Autodesk Inventor part; units mm, degrees
ref_plane "YZ Plane" through (0, 0, 0) normal (1, 0, 0) x (0, 1, 0)
ref_plane "XZ Plane" through (0, 0, 0) normal (0, 1, 0) x (-1, 0, 0)
ref_plane "XY Plane" through (0, 0, 0) normal (0, 0, 1) x (1, 0, 0)
sketch "Sketch1" plane through (0, 0, 0) normal (0, 0, 1) x (1, 0, 0)
  line L0 (0, 0) -> (103.9622, 0)
  line L1 (103.9622, 0) -> (103.9622, 50.8)
  line L2 (103.9622, 50.8) -> (0, 50.8)
  line L3 (0, 50.8) -> (0, 0)
  line L4 (0, 50.8) -> (103.9622, 50.8)
  line L5 (103.9622, 50.8) -> (103.9622, 42.9936)
  line L6 (0, 42.9936) -> (0, 50.8)
  dimension "d4" = 103.9622
  dimension "d5" = 50.8
extrude "Extrusion1" add sketch "Sketch1" along normal blind 2.54
sketch "Sketch6" plane through (0, 0, 2.54) normal (0, 0, 1) x (1, 0, 0)
  line L0 (103.9622, 0) -> (103.9622, 50.8)
  line L1 (103.9622, 50.8) -> (0, 50.8)
  line L2 (0, 50.8) -> (0, 0)
  line L3 (0, 0) -> (103.9622, 0)
  line L4 (0, 0) -> (2.54, 0)
  line L5 (2.54, 0) -> (2.54, 50.8)
  line L6 (2.54, 50.8) -> (0, 50.8)
  line L7 (0, 50.8) -> (0, 0)
  dimension "d23" = 2.54
  dimension "d24" = 50.8
extrude "Extrusion5" add sketch "Sketch6" along normal blind 103.9622 contours L3 L2 L1 L5
sketch "Sketch7" plane through (2.54, 0, 2.54) normal (1, 0, 0) x (0, 0, -1)
  line L0 (0, 50.8) -> (0, 0)
  line L1 (0, 50.8) -> (-103.9622, 50.8)
  line L2 (-103.9622, 0) -> (-103.9622, 50.8)
  line L3 (0, 0) -> (-103.9622, 0)
  line L4 (2.54, 0) -> (2.54, 50.8)
  line L5 (2.54, 50.8) -> (0, 50.8)
  line L6 (0, 0) -> (0, 50.8)
  line L7 (2.54, 0) -> (0, 0)
  line L8 (0, 50.8) -> (0, 0)
  line L9 (0, 50.8) -> (-103.9622, 50.8)
  line L10 (-103.9622, 0) -> (-103.9622, 50.8)
  line L11 (0, 0) -> (-103.9622, 0)
  circle A0 centre (-10.2616, 39.1541) radius 1.905
  circle A1 centre (-10.2616, 11.6459) radius 1.905
  circle A2 centre (-54.7116, 39.1541) radius 1.905
  circle A3 centre (-54.7116, 11.6459) radius 1.905
  dimension "d27" = 3.81
  dimension "d28" = 11.6459
  dimension "d29" = 10.2616
  dimension "d30" = 3.81
  dimension "d31" = 11.6459
  dimension "d32" = 3.81
  dimension "d33" = 3.81
  dimension "d34" = 44.45
  dimension "d35" = 44.45
  dimension "d36" = 11.6459
  dimension "d37" = 10.2616
  dimension "d38" = 11.6459
extrude "Extrusion6" cut sketch "Sketch7" against normal through all contours A0 | A1 | A2 | A3
sketch "Sketch8" plane through (0, 0, 2.54) normal (0, 0, 1) x (1, 0, 0)
  circle A0 centre (12.8016, 39.1541) radius 1.905
  circle A1 centre (12.8016, 11.6459) radius 1.905
  circle A2 centre (57.2516, 39.1541) radius 1.905
  circle A3 centre (57.2516, 11.6459) radius 1.905
  line L0 (103.9622, 50.8) -> (2.54, 50.8)
  line L1 (2.54, 0) -> (103.9622, 0)
  line L2 (2.54, 0) -> (2.54, 50.8)
  line L3 (103.9622, 50.8) -> (26.416, 50.8)
  line L4 (26.416, 50.8) -> (26.416, 48.26)
  line L5 (26.416, 48.26) -> (103.9622, 48.26)
  line L6 (103.9622, 48.26) -> (103.9622, 50.8)
  line L7 (2.54, 13.5509) -> (2.54, 9.7409)
  line L8 (2.54, 41.0591) -> (2.54, 37.2491)
  line L9 (2.54, 13.5509) -> (2.54, 9.7409)
  line L10 (2.54, 41.0591) -> (2.54, 37.2491)
  line L11 (2.54, 50.8) -> (2.54, 0)
  line L12 (2.54, 0) -> (2.54, 50.8)
  line L13 (2.54, 13.5509) -> (2.54, 9.7409)
  line L14 (2.54, 41.0591) -> (2.54, 37.2491)
  line L15 (2.54, 13.5509) -> (2.54, 9.7409)
  line L16 (2.54, 41.0591) -> (2.54, 37.2491)
  line L17 (2.54, 50.8) -> (2.54, 0)
  line L18 (2.54, 0) -> (2.54, 50.8)
  point P0 (0, 0)
  dimension "d41" = 3.81
  dimension "d42" = 3.81
  dimension "d43" = 3.81
  dimension "d44" = 3.81
  dimension "d45" = 11.6459
  dimension "d46" = 11.6459
  dimension "d47" = 11.6459
  dimension "d48" = 11.6459
  dimension "d49" = 10.2616
  dimension "d50" = 10.2616
  dimension "d51" = 44.45
  dimension "d52" = 44.45
  dimension "d55" = 77.5462
  dimension "d56" = 2.54
extrude "Extrusion7" cut sketch "Sketch8" against normal through all contours A0 | A1 | A2 | A3
sketch "Sketch9" plane through (2.54, 0, 2.54) normal (1, 0, 0) x (0, 0, -1)
  circle A0 centre (-54.7116, 11.6459) radius 1.905
  circle A1 centre (-54.7116, 39.1541) radius 1.905
  circle A2 centre (-10.2616, 11.6459) radius 1.905
  circle A3 centre (-10.2616, 39.1541) radius 1.905
  line L0 (0, 50.8) -> (0, 0)
  line L1 (0, 50.8) -> (-103.9622, 50.8)
  line L2 (-103.9622, 0) -> (-103.9622, 50.8)
  line L3 (0, 0) -> (-103.9622, 0)
  line L4 (-103.9622, 50.8) -> (-26.416, 50.8)
  line L5 (-26.416, 50.8) -> (-26.416, 48.26)
  line L6 (-26.416, 48.26) -> (-103.9622, 48.26)
  line L7 (-103.9622, 48.26) -> (-103.9622, 50.8)
  point P0 (2.54, 0)
  point P1 (-26.416, 50.8)
  dimension "d57" = 77.5462
  dimension "d58" = 2.54
extrude "Extrusion8" add sketch "Sketch9" along normal blind 16.129 contours L5 L6 L2 L1
sketch "Sketch10" plane through (0, 0, 2.54) normal (0, 0, 1) x (1, 0, 0)
  circle A0 centre (12.8016, 11.6459) radius 1.905
  circle A1 centre (57.2516, 39.1541) radius 1.905
  circle A2 centre (57.2516, 11.6459) radius 1.905
  circle A3 centre (12.8016, 39.1541) radius 1.905
  line L0 (2.54, 50.8) -> (2.54, 0)
  line L1 (2.54, 0) -> (103.9622, 0)
  line L2 (103.9622, 0) -> (103.9622, 50.8)
  line L3 (103.9622, 50.8) -> (2.54, 50.8)
  line L4 (103.9622, 50.8) -> (26.416, 50.8)
  line L5 (26.416, 50.8) -> (26.416, 48.26)
  line L6 (26.416, 48.26) -> (103.9622, 48.26)
  line L7 (103.9622, 48.26) -> (103.9622, 50.8)
  point P0 (0, 0)
  dimension "d61" = 77.5462
  dimension "d62" = 2.54
extrude "Extrusion9" add sketch "Sketch10" along normal blind 16.129 contours L3 L2 L6 L5
sketch "Sketch11" plane through (0, 50.8, 0) normal (0, 1, 0) x (1, 0, 0)
  line L0 (103.9622, 0) -> (0, 0)
  line L1 (0, 0) -> (0, -106.5022)
  line L2 (0, -106.5022) -> (18.669, -106.5022)
  line L3 (18.669, -28.956) -> (18.669, -106.5022)
  line L4 (2.54, -28.956) -> (18.669, -28.956)
  line L5 (2.54, -2.54) -> (2.54, -28.956)
  line L6 (26.416, -2.54) -> (2.54, -2.54)
  line L7 (26.416, -2.54) -> (26.416, -18.669)
  line L8 (103.9622, -18.669) -> (26.416, -18.669)
  line L9 (103.9622, 0) -> (103.9622, -18.669)
  line L10 (15.0876, -28.956) -> (15.0876, -106.5022)
  circle A0 centre (15.0876, -93.8022) radius 2.5019
  circle A1 centre (15.0876, -81.1022) radius 2.5019
  circle A2 centre (15.0876, -68.4022) radius 2.5019
  circle A3 centre (15.0876, -55.7022) radius 2.5019
  circle A4 centre (15.0876, -43.0022) radius 2.5019
  line L11 (26.416, -15.0876) -> (103.9622, -15.0876)
  circle A5 centre (91.2622, -15.0876) radius 2.5019
  circle A6 centre (78.5622, -15.0876) radius 2.5019
  circle A7 centre (65.8622, -15.0876) radius 2.5019
  circle A8 centre (53.1622, -15.0876) radius 2.5019
  circle A9 centre (40.4622, -15.0876) radius 2.5019
  point P0 (0, 0)
  dimension "d65" = 3.5814
  dimension "d66" = 5.0038
  dimension "d67" = 12.7
  dimension "d70" = 12.7
  dimension "d75" = 3.5814
  dimension "d76" = 5.0038
  dimension "d77" = 12.7
  dimension "d80" = 12.7
extrude "Extrusion10" cut sketch "Sketch11" against normal blind 16.129 contours A5 L11 | L11 A5 | A0 L10 | L10 A0 | A6 L11 | L11 A6 | A9 L11 | L11 A9 | A1 L10 | L10 A1 | A7 L11 | L11 A7 | A4 L10 | L10 A4 | A8 L11 | L11 A8 | A2 L10 | L10 A2 | A3 L10 | L10 A3
properties part number "BDVBS_002_Brachet 2" material "Aluminum 6061"
Model file for the job. Use its own axes, mm. A direction names the side the tool comes from. Give positions to 0.01 mm unless a question says otherwise; leave off trailing zeros. Loops run counter-clockwise (first coordinate to the right, second up) from the corner with the lowest first, then second, coordinate; pieces in that order, holes last. Notation, with made-up numbers: (-20.5, -18.5) -> (8.5, -18.5) arc R23 ccw to (8.5, 15.5) -> close; hole circle Ø2 at (-2, 51). An arc over 180 degrees is marked (long way). Write each question's results on one line, items separated by ' | '.
(1) Probe line 1 along X through (y, z) = (27.5, 33); line 2 along Y through (x, z) = (13, 35). List the from-to ranges inside material, lowest first.
Geometry results:
line 1: x = 0 to 2.54 | line 2: y = 48.26 to 50.8
(2) Cut at C-C on x = 23.5. List the corners of the cut face in (y, z).
Geometry results:
outline: (0, 0) -> (50.8, 0) -> (50.8, 2.54) -> (0, 2.54) -> close
(3) Cut at B-B on z = 34. List the corners of the cut face in (x, y), and give its area (3 significant figures).
Geometry results:
outline: (0, 0) -> (2.54, 0) -> (2.54, 48.26) -> (18.67, 48.26) -> (18.67, 50.8) -> (0, 50.8) -> close | area: 170 mm²
(4) Tool access for faces 1 (the cylindrical face through (1.288, 13.535, 13.05)), 2 (the flat face through (18.669, 50, 68)), 3 (the flat face through (65, 48.26, 10)): list every direction of +Z, -Z, +X, -X, +Y, -Y with a clear straight run to the whole face (end or side of a thin tool).
Geometry results:
face 1: +X, -X | face 2: +Z, +X, +Y, -Y | face 3: +Z, +X, -Y
(5) Flat gauge pins, fed straight in: pin 1 Ø8 at (x, z) = (65.86, 15.09) entering from -Y; pin 2 Ø2 at (x, y) = (59.5, 49.5) entering from +Z; pin 3 Ø1 at (x, y) = (74, 44.5) entering from +Z. Where does each tip first touch, or does it go through?
Geometry results:
pin 1: stops at y = 48.26 | pin 2: stops at z = 18.67 | pin 3: stops at z = 2.54
(6) Cut at A-A on y = 35.5. List the corners of the cut face in (x, z).
Geometry results:
outline: (0, 0) -> (103.96, 0) -> (103.96, 2.54) -> (2.54, 2.54) -> (2.54, 106.5) -> (0, 106.5) -> close
(7) Pull direction Z, two halves, no side cores. Call faces 4 (the cylindrical face through (14.76, 49.55, 78.62)), 5 (the flat face through (65, 50, 18.669)), 6 (the cylindrical face through (12.389, 37.294, 1.288)): released by +Z, released by -Z, zero draft, split by the parting line, or undercut.
Geometry results:
face 4: undercut | face 5: released by +Z | face 6: zero draft
